CAD build for the part. Positions are in the model's coordinates, mm. A direction names the side the tool comes from. Round coordinates to 2 decimals unless told otherwise and drop trailing zeros. Loops run counter-clockwise (first coordinate to the right, second up) from the corner with the lowest first, then second, coordinate; pieces in that order, holes last. Notation, with made-up numbers: (-20.75, 4.5) - (30.25, 4.5) arc R24 cw to (30.25, 34.5) - close; hole circle Ø11 at (39, 42.5). An arc over 180 degrees is marked (long way). Use one line per item in the form item = value.
Autodesk Inventor part; units mm, degrees
ref_plane "YZ Plane" through (0, 0, 0) normal (1, 0, 0) x (0, 1, 0)
ref_plane "XZ Plane" through (0, 0, 0) normal (0, 1, 0) x (-1, 0, 0)
ref_plane "XY Plane" through (0, 0, 0) normal (0, 0, 1) x (1, 0, 0)
sketch "Sketch1" plane through (0, 0, 0) normal (0, 1, 0) x (-1, 0, 0)
  line L0 (0, 0) -> (44, 0)
  line L1 (44, 0) -> (44, -300)
  line L2 (44, -300) -> (0, -300)
  line L3 (0, -300) -> (0, 0)
  dimension "d0" = 300
  dimension "d1" = 44
extrude "Extrusion1" add sketch "Sketch1" along normal blind 20
sketch "Sketch2" plane through (-44, 0, 0) normal (0, 0, 1) x (1, 0, 0)
  line L0 (44, 20) -> (0, 20)
  line L1 (44, 0) -> (0, 0)
  line L2 (0, 0) -> (44, 0)
  line L3 (44, 0) -> (44, 22)
  line L4 (44, 22) -> (0, 22)
  line L5 (0, 22) -> (0, 0)
  circle A0 centre (22, 22) radius 20.5
  dimension "d17" = 22
  dimension "d18" = 41
  dimension "d19" = 22
extrude "Extrusion2" cut sketch "Sketch2" against normal up to surface (300 mm away) contours A0 L0 | L0 A0 L4 | L4 A0
sketch "Sketch3" plane through (-44, 0, 0) normal (0, 0, 1) x (1, 0, 0)
  line L0 (0, 0) -> (0, 20)
  line L1 (0, 20) -> (44, 20)
  line L2 (44, 20) -> (44, 0)
  line L3 (44, 0) -> (0, 0)
  line L4 (0, 0) -> (0, 20)
extrude "Extrusion3" add sketch "Sketch3" against normal blind 5
sketch "Sketch4" plane through (0, 0, -300) normal (0, 0, -1) x (-1, 0, 0)
  line L0 (0, 0) -> (0, 20)
  line L1 (44, 0) -> (0, 0)
  line L2 (0, 20) -> (44, 20)
  line L3 (44, 20) -> (44, 0)
  line L4 (44, 0) -> (0, 0)
  line L5 (0, 0) -> (0, 20)
extrude "Extrusion4" add sketch "Sketch4" against normal blind 5
chamfer "Chamfer1" distance 4 angle 45 1 edges at (0, 0, -150)
chamfer "Chamfer2" distance 4 angle 45 1 edges at (-44, 0, -150)
sketch "Sketch5" plane through (0, 20, -300) normal (0, 0, -1) x (-1, 0, 0)
  line L0 (0, 0) -> (44, 0)
  line L1 (44, 0) -> (44, -20)
  line L2 (44, -20) -> (0, -20)
  line L3 (0, -20) -> (0, 0)
  line L4 (44, -16) -> (40, -20)
  line L5 (4, -20) -> (0, -16)
  line L6 (22, 0) -> (22, -20)
  line L7 (0, -10) -> (44, -10)
  line L8 (11.8539, 0) -> (11.8539, -20)
  line L9 (32.3539, 0) -> (32.3539, -20)
  line L10 (10.8539, 0) -> (10.8539, -20)
  line L11 (33.3539, 0) -> (33.3539, -20)
  line L12 (0, -9) -> (44, -9)
  circle A0 centre (11.8539, 0) radius 2
  circle A1 centre (32.3539, 0) radius 2
  point P0 (0, -20)
  point P1 (2, -18)
  point P2 (42, -18)
  point P3 (11.8539, -2)
  point P4 (10.8539, -1.7321)
  point P5 (10.8539, -10)
  point P6 (33.3539, -10)
  point P7 (33.3539, -1.7321)
  point P8 (32.3539, -2)
  point P9 (32.3539, -9)
  point P10 (11.8539, -9)
  dimension "d20" = 20
  dimension "d21" = 44
  dimension "d23" = 2
  dimension "d24" = 2
  dimension "d25" = 20.5
  dimension "d26" = 11.8539
  dimension "d27" = 1
  dimension "d28" = 1
  dimension "d29" = 9
  dimension "d30" = 4
  dimension "d31" = 4
extrude "Extrusion5" add sketch "Sketch5" along normal blind 2.5 contours A0 L8 L12 L10 | L12 L8 L7 L10 | L12 L6 L7 L8 | L12 L9 L7 L6 | A1 L11 L12 L9 | L12 L11 L7 L9
sketch "Sketch7" plane through (-33.3539, 10, -300) normal (0, -1, 0) x (1, 0, 0)
  line L0 (22.5, -2.5) -> (0, -2.5)
  line L1 (0, -2.5) -> (0, -4)
  line L2 (0, -4) -> (22.5, -4)
  line L3 (22.5, -4) -> (22.5, -2.5)
  line L4 (0, 0) -> (0, -2.5)
  line L5 (22.5, -4) -> (21.5, -4)
  line L6 (21.5, -2.5) -> (22.5, -2.5)
  line L7 (22.5, -2.5) -> (22.5, -4)
  line L8 (21.5, 0) -> (21.5, -2.5)
  line L9 (3, -2.5) -> (0, -2.5)
  line L10 (0, -2.5) -> (0, -4)
  line L11 (0, -4) -> (3, -4)
  line L12 (3, -4) -> (3, -2.5)
  line L13 (22.5, -2.5) -> (0, -2.5)
  line L14 (22.5, -4) -> (19.5, -4)
  line L15 (19.5, -4) -> (19.5, -2.5)
  line L16 (19.5, -2.5) -> (22.5, -2.5)
  line L17 (22.5, -2.5) -> (22.5, -4)
  point P0 (33.3539, 300)
  point P1 (22.5, -3.25)
  point P2 (19.5, -4)
  point P3 (19.5, -2.5)
  point P4 (3, -4)
  dimension "d36" = 1.5
  dimension "d37" = 3
  dimension "d38" = 3
extrude "Extrusion6" add sketch "Sketch7" against normal blind 3 contours L15 L2 L12 L0
extrude "Extrusion7" add sketch "Sketch7" against normal blind 9 contours L3 L2 L15 L0 | L12 L2 L1 L0
properties part number "profilrampa"
1) Two-plate mould, pull along Z, no slides. Class faces 4 (the flat face through (-22, 10, 0)), 5 (the flat face through (-22, 12, -302.5)), 6 (the flat face through (-44, 12, -148)): +Z half, -Z half, draft (parallel to the pull), parting line (faces both ways), or undercut.
Report:
face_4 = +Z half
face_5 = undercut
face_6 = draft
2) Drill centre lines: probe 1 along Z at (x, y) = (-24, 11.5); probe 2 along Z at (x, y) = (-38, 13); probe 3 along X at (y, z) = (16.5, -206). Where is each one in solid material? Low to high.
Report:
probe_1 = -304 to -302.5, -300 to -295, -5 to 0
probe_2 = -300 to -295, -5 to 0
probe_3 = -44 to -41.75, -2.25 to 0
3) Flat gauge pins, fed straight in: pin 1 (1.2 mm diameter, centred on x = -24, z = -303, fed in from -Y); pin 2 (2 mm diameter, centred on x = -35.5, z = -94.5, fed in from +Y); pin 3 (2 mm diameter, centred on y = 15.5, z = -301.5, fed in from +X). Where does each tip first touch, or does it go through?
Report:
pin_1 = 10
pin_2 = 7.51
pin_3 = -10.85
4) Slice it at B-B (z = -143.5). Write the cut outline in (x, y).
Report:
outline = (-44, 4) - (-40, 0) - (-4, 0) - (0, 4) - (0, 20) - (-1.6, 20) arc R20.5 cw to (-42.4, 20) - (-44, 20) - close
5) Tool access for faces 1 (the flat face through (-22, 13, -295)), 2 (the flat face through (-22, 12, -304)), 3 (the flat face through (-22, 12, -300)): list every direction of +Z, -Z, +X, -X, +Y, -Y with a clear straight run to the whole face (end or side of a thin tool).
Report:
face_1 = +Y
face_2 = -Z, +X, -X, +Y, -Y
face_3 = none
6) Slice it at A-A (y = 15.5). Write the cut outline in (x, z), plus the area to 3 significant figures.
Report:
outline = (-44, -300) - (-33.35, -300) - (-33.35, -304) - (-30.35, -304) - (-30.35, -302.5) - (-32.35, -302.5) - (-32.35, -300) - (-11.85, -300) - (-11.85, -302.5) - (-13.85, -302.5) - (-13.85, -304) - (-10.85, -304) - (-10.85, -300) - (0, -300) - (0, 0) - (-44, 0) - close; hole (-41.44, -295) - (-2.56, -295) - (-2.56, -5) - (-41.44, -5) - close
area = 1,940 mm^2
7) Slice it at C-C (x = -20.5). Write the cut outline in (y, z), plus the area to 3 significant figures.
Report:
outline = (0, -300) - (10, -300) - (10, -304) - (13, -304) - (13, -302.5) - (11, -302.5) - (11, -300) - (20, -300) - (20, -295) - (1.55, -295) - (1.55, -5) - (20, -5) - (20, 0) - (0, 0) - close
area = 658 mm^2
